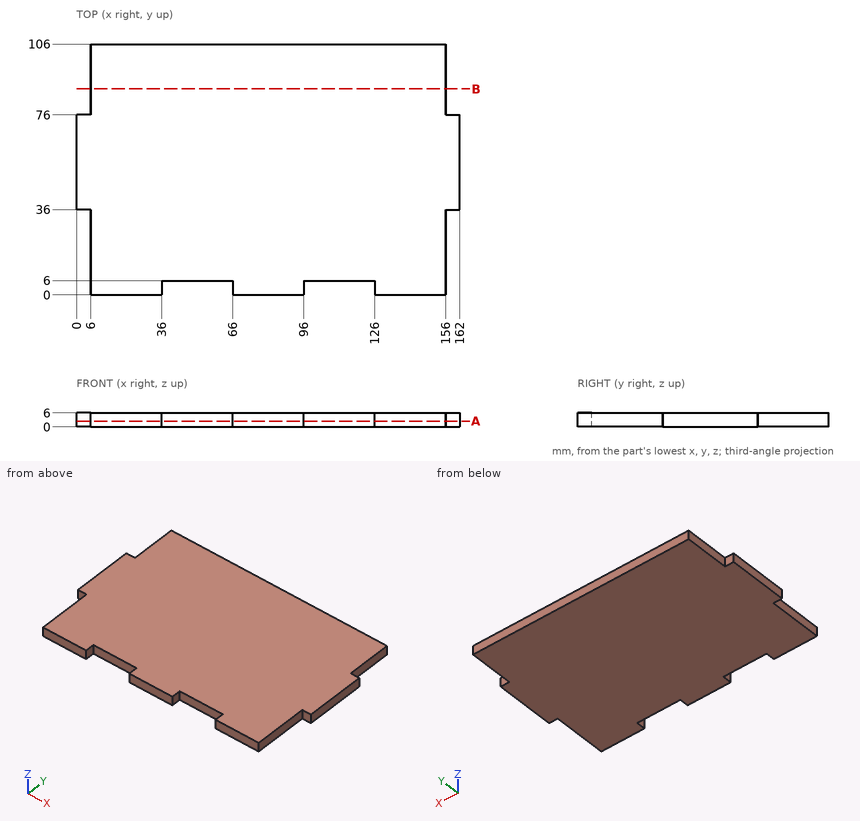
The figure shows three views and two pictorial views of one solid part (mm, origin at its lowest corner). Answer the questions. Coordinates: 2 decimals unless noted, no trailing zeros. Loops run counter-clockwise (first coordinate to the right, second up) from the corner with the lowest first, then second, coordinate; pieces in that order, holes last.
(1) Consider line 1 along X through (y, z) = (4, 3); line 2 along Y through (x, z) = (110, 1.65); line 3 along X through (y, z) = (93.5, 5.2). Determine where each line is inside the solid, lowest interval first.
Solution:
line 1: x = 6 to 36, 66 to 96, 126 to 156
line 2: y = 6 to 106
line 3: x = 6 to 156
(2) Flat-ended cylindrical pins translate along their axes: pin 1 Ø3 at (y, z) = (2.5, 1.5) entering from -X; pin 2 Ø1.8 at (y, z) = (10, 3) entering from +X; pin 3 Ø1.8 at (x, z) = (108.5, 1.5) entering from -Y. Find the tip coordinate at first contact, or state that the pin passes through.
Solution:
pin 1: stops at x = 6
pin 2: stops at x = 156
pin 3: stops at y = 6
(3) The part is cut by section B-B (y = 87). Determine the outline of the cut face in (x, z), and give its area (3 significant figures).
Solution:
outline: (6, 0) - (156, 0) - (156, 6) - (6, 6) - close
area: 900 mm2
(4) The part is cut by section A-A (z = 2.45). Determine the outline of the cut face in (x, y).
Solution:
outline: (0, 36) - (6, 36) - (6, 0) - (36, 0) - (36, 6) - (66, 6) - (66, 0) - (96, 0) - (96, 6) - (126, 6) - (126, 0) - (156, 0) - (156, 36) - (162, 36) - (162, 76) - (156, 76) - (156, 106) - (6, 106) - (6, 76) - (0, 76) - close
